Can you work these out from the model? Positions are in its coordinate system, mm. Face numbers are marked on the shaded views. A direction names the side the tool comes from. Give positions to 0.01 mm unless a question says otherwise; leave off trailing zeros. Loops run counter-clockwise (first coordinate to the right, second up) from the corner with the lowest first, then second, coordinate; pieces in that order, holes last.
from build123d import *

# Parameters (mm, degrees)
RESSALTO_EXTRUS_O1_DEPTH   = 160
ESBO_O2_W                  = 7.6
ESBO_O2_H                  = 120
CORTE_EXTRUS_O1_DEPTH      = 30
CORTE_EXTRUS_O2_DEPTH      = 30
F_3DSKETCH3_R              = 2
CORTE_EXTRUS_O3_DEPTH      = 70
ESBO_O3_W                  = 45.015344868
ESBO_O3_H                  = 129.478543367
ESBO_O3_W_2                = 37.192593828
CORTE_EXTRUS_O4_DEPTH      = 31.510345968
CORTE_EXTRUS_O4_DEPTH_BACK = 38
ESBO_O4_R                  = 12
CORTE_EXTRUS_O5_DEPTH      = 52.510345968
CORTE_EXTRUS_O5_DEPTH_BACK = 54
ESBO_O5_R                  = 15.084668413
ESBO_O5_R_2                = 12
RESSALTO_EXTRUS_O3_DEPTH   = 9


with BuildPart() as part:
    # Esboço1 → Ressalto-extrusão1 (new body)
    with BuildSketch(Plane.XY):
        with BuildLine():
            Line((-3.8, 21.821375341), (-3.8, -98.178624659))
            Line((-3.8, -98.178624659), (-5.7, -98.178624659))
            Line((-5.7, -98.178624659), (-5.360626179, -99.63308389))
            ThreePointArc((-5.360626179, -99.63308389), (-4.656141559, -100.745296045), (-3.41294376, -101.178624659))
            Line((-3.41294376, -101.178624659), (3.41294376, -101.178624659))
            ThreePointArc((3.41294376, -101.178624659), (4.656141559, -100.745296045), (5.360626179, -99.63308389))
            Line((5.360626179, -99.63308389), (5.7, -98.178624659))
            Line((5.7, -98.178624659), (3.8, -98.178624659))
            Line((3.8, -98.178624659), (3.8, 21.821375341))
            Line((3.8, 21.821375341), (5.7, 21.821375341))
            Line((5.7, 21.821375341), (4.013268169, 24.033911877))
            ThreePointArc((4.013268169, 24.033911877), (3.310139149, 24.613730366), (2.422747768, 24.821375341))
            Line((2.422747768, 24.821375341), (-2.297792791, 24.821375341))
            ThreePointArc((-2.297792791, 24.821375341), (-3.27177376, 24.568189891), (-3.999156919, 23.872736414))
            Line((-3.999156919, 23.872736414), (-5.266799243, 21.821375341))
            Line((-5.266799243, 21.821375341), (-3.8, 21.821375341))
        make_face()
    extrude(amount=RESSALTO_EXTRUS_O1_DEPTH)

    # Esboço2 → Corte-extrusão1 (cut)
    with BuildSketch(Plane.XY):
        with Locations((0, -38.178624659)):
            Rectangle(ESBO_O2_W, ESBO_O2_H)
    extrude(amount=CORTE_EXTRUS_O1_DEPTH, mode=Mode.SUBTRACT)

    # 3DSketch2 → Corte-extrusão2 (cut)
    with BuildSketch(Plane(origin=(-3.8, 21.821375341, 160), x_dir=(0.0632066956560733, -0.9980004577274705, 0), z_dir=(0, 0, -1))):
        Polygon((0, 0), (0.480370887, -7.584803479), (120.240425814, 0), (119.760054927, 7.584803479), align=None)
    extrude(amount=CORTE_EXTRUS_O2_DEPTH, mode=Mode.SUBTRACT)

    # 3DSketch3 → Corte-extrusão3 (cut)
    with BuildSketch(Plane(origin=(3.8, -38.178624659, 80), x_dir=(0, 0.7676852805184269, 0.6408270516101394), z_dir=(1, 0, 0))):
        with Locations(Location((0, 0, 0), (0, 0, 140.146481665))):
            Circle(F_3DSKETCH3_R)
        with Locations(Location((23.030558416, -19.224811548, 0), (0, 0, 140.146481665))):
            Circle(F_3DSKETCH3_R)
        with Locations(Location((-23.030558416, 19.224811548, 0), (0, 0, 140.146481665))):
            Circle(F_3DSKETCH3_R)
        with Locations(Location((-39.051234706, 0.032679535, 0), (0, 0, 140.146481665))):
            Circle(F_3DSKETCH3_R)
        with Locations(Location((-16.02067629, -19.192132013, 0), (0, 0, 140.146481665))):
            Circle(F_3DSKETCH3_R)
        with Locations(Location((7.009882125, -38.416943561, 0), (0, 0, 140.146481665))):
            Circle(F_3DSKETCH3_R)
        with Locations(Location((-6.982602808, 38.449623097, 0), (0, 0, 140.146481665))):
            Circle(F_3DSKETCH3_R)
        with Locations(Location((16.047955607, 19.224811548, 0), (0, 0, 140.146481665))):
            Circle(F_3DSKETCH3_R)
        with Locations(Location((39.078514023, 0, 0), (0, 0, 140.146481665))):
            Circle(F_3DSKETCH3_R)
    extrude(amount=-CORTE_EXTRUS_O3_DEPTH, mode=Mode.SUBTRACT)

    # Esboço3 → Corte-extrusão4 (cut, two sides)
    with BuildSketch(Plane(origin=(0, 0, 0), x_dir=(0, 0, -1), z_dir=(1, 0, 0))) as corte_extrus_o4_sk:
        with Locations((-7.492327566, -39.917896343)):
            Rectangle(ESBO_O3_W, ESBO_O3_H)
        with Locations((-148.596296914, -39.917896343)):
            Rectangle(ESBO_O3_W_2, ESBO_O3_H)
    extrude(amount=CORTE_EXTRUS_O4_DEPTH, mode=Mode.SUBTRACT)
    extrude(corte_extrus_o4_sk.sketch, amount=-CORTE_EXTRUS_O4_DEPTH_BACK, mode=Mode.SUBTRACT)

    # Esboço4 → Corte-extrusão5 (cut, two sides)
    with BuildSketch(Plane(origin=(0, 0, 0), x_dir=(0, 0, -1), z_dir=(1, 0, 0))) as corte_extrus_o5_sk:
        with Locations(Location((-80, -38.178624659, 0), (0, 0, 270))):
            Circle(ESBO_O4_R)
    extrude(amount=CORTE_EXTRUS_O5_DEPTH, mode=Mode.SUBTRACT)
    extrude(corte_extrus_o5_sk.sketch, amount=-CORTE_EXTRUS_O5_DEPTH_BACK, mode=Mode.SUBTRACT)

    # Esboço5 → Ressalto-extrusão3 (add)
    with BuildSketch(Plane(origin=(0, 0, 0), x_dir=(0, 0, -1), z_dir=(1, 0, 0))):
        with Locations(Location((-80, -38.178624659, 0), (0, 0, 270))):
            Circle(ESBO_O5_R)
        with Locations((-80, -38.178624659)):
            Circle(ESBO_O5_R_2, mode=Mode.SUBTRACT)
    extrude(amount=RESSALTO_EXTRUS_O3_DEPTH)


solid = part.part
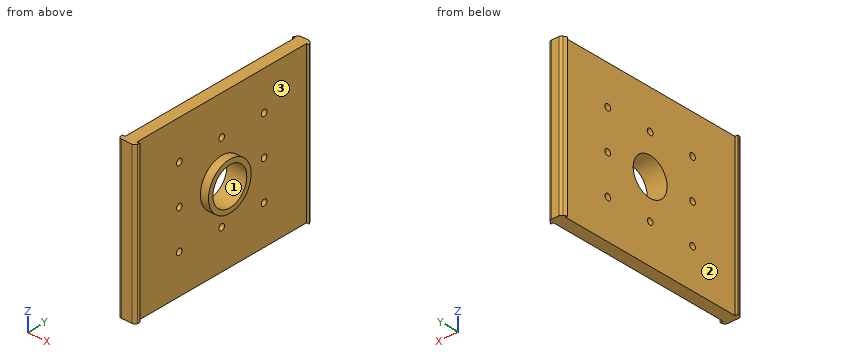
(1) Will these pins go through, and if not, where does the flat tip stop? P1, Ø8, axis at y = 9, z = 89.5, coming from the +X side; P2, Ø1.2, axis at x = -4.5, z = 64, coming from the -Y side; P3, Ø2, axis at y = -55, z = 103, coming from the -X side.
Returned:
P1: stops at x = 3.8
P2: stops at y = -101.12
P3: stops at x = -3.8
(2) Suppose I cut it at D-D on z = 90. List the corners of the cut face in (x, y) for me.
Returned:
outline: (-5.7, -98.18) - (-5.36, -99.63) arc R2 ccw to (-3.41, -101.18) - (3.41, -101.18) arc R2 ccw to (5.36, -99.63) - (5.7, -98.18) - (3.8, -98.18) - (3.8, -49.47) - (9, -49.47) - (9, -44.81) - (-3.8, -44.81) - (-3.8, -98.18) - close; (-5.27, 21.82) - (-3.8, 21.82) - (-3.8, -31.55) - (9, -31.55) - (9, -26.88) - (3.8, -26.88) - (3.8, 21.82) - (5.7, 21.82) - (4.01, 24.03) arc R2 ccw to (2.42, 24.82) - (-2.3, 24.82) arc R2 ccw to (-4, 23.87) - close
(3) Which directions (+Z, -Z, +X, -X, +Y, -Y) give clear straight access to the entire face, cutting with the end or side of a thin tool? Please do the marked faces 1, 2 and 3.
Returned:
face 1: +X, -X
face 2: +Z, -Z, -X
face 3: +X
(4) Suppose I cut it at C-C on x = -0.5. Give the number of separate pieces and of enclosed holes in the cut face, plus the area to 3 significant figures.
Returned:
separate pieces: 1
enclosed holes: 9
area: 12,000 mm2
(5) Please list where these lines run through material, in increasing order: probe 1 along Z at (x, y) = (-1, -38); probe 2 along Y at (x, z) = (4.25, 80); probe 3 along X at (y, z) = (-78, 47).
Returned:
probe 1: z = 30 to 53.01, 56.99 to 68, 92 to 103.05, 107.03 to 130
probe 2: y = -101 to -98.18, -53.26 to -50.18, -26.18 to -23.09, 21.82 to 23.72
probe 3: x = -3.8 to 3.8
(6) Suppose I cut it at B-B on y = -31.5. List the corners of the cut face in (x, z) for me, plus the area to 3 significant figures.
Returned:
outline: (-3.8, 30) - (3.8, 30) - (3.8, 66.47) - (9, 66.47) - (9, 70.03) - (-3.8, 70.03) - close; (-3.8, 89.97) - (9, 89.97) - (9, 93.53) - (3.8, 93.53) - (3.8, 130) - (-3.8, 130) - close
area: 645 mm2
(7) Suppose I cut it at A-A on z = 55. List the corners of the cut face in (x, y) for me.
Returned:
outline: (-5.7, -98.18) - (-5.36, -99.63) arc R2 ccw to (-3.41, -101.18) - (3.41, -101.18) arc R2 ccw to (5.36, -99.63) - (5.7, -98.18) - (3.8, -98.18) - (3.8, -70.18) - (-3.8, -70.18) - (-3.8, -98.18) - close; (-5.27, 21.82) - (-3.8, 21.82) - (-3.8, -6.18) - (3.8, -6.18) - (3.8, 21.82) - (5.7, 21.82) - (4.01, 24.03) arc R2 ccw to (2.42, 24.82) - (-2.3, 24.82) arc R2 ccw to (-4, 23.87) - close; (-3.8, -66.18) - (3.8, -66.18) - (3.8, -40.18) - (-3.8, -40.18) - close; (-3.8, -36.18) - (3.8, -36.18) - (3.8, -10.18) - (-3.8, -10.18) - close
